```python
from build123d import *

# Parameters (mm, degrees)
F1_DEPTH = 6


with BuildPart() as f1:
    # F0 (on Right) → F1 (new body)
    with BuildSketch(Plane.YZ):
        Polygon((62.5, 142.2184194922), (9.4337919727, 142.2184194922), (9.4337919727, 134.7184194922), (47.5, 134.7184194922), (47.5, 129.8368871212), (62.5, 129.8368871212), align=None)
        Polygon((9.4337919727, 142.2184194922), (-47.5, 142.2184194922), (-47.5, -47.7815805078), (62.5, -47.7815805078), (62.5, 129.8368871212), (47.5, 129.8368871212), (47.5, 114.7184194922), (-32.5, 114.7184194922), (-32.5, 134.7184194922), (9.4337919727, 134.7184194922), align=None)
        Polygon((-22.5, -4.2815805078), (-22.5, -7.7815805078), (-22.5, -11.2815805078), (-32.5, -11.2815805078), (-32.5, -4.2815805078), align=None, mode=Mode.SUBTRACT)
        Polygon((12.5, -4.2815805078), (12.5, -7.7815805078), (12.5, -11.2815805078), (2.5, -11.2815805078), (2.5, -7.7815805078), (2.5, -4.2815805078), align=None, mode=Mode.SUBTRACT)
        Polygon((37.5, -7.7815805078), (37.5, -4.2815805078), (47.5, -4.2815805078), (47.5, -11.2815805078), (37.5, -11.2815805078), align=None, mode=Mode.SUBTRACT)
        Polygon((-22.5, 55.7184194922), (-22.5, 52.2184194922), (-22.5, 48.7184194922), (-32.5, 48.7184194922), (-32.5, 55.7184194922), align=None, mode=Mode.SUBTRACT)
        Polygon((-22.5, 101.2184194922), (-22.5, 97.7184194922), (-32.5, 97.7184194922), (-32.5, 104.7184194922), (-22.5, 104.7184194922), align=None, mode=Mode.SUBTRACT)
        Polygon((12.5, 55.7184194922), (12.5, 52.2184194922), (12.5, 48.7184194922), (2.5, 48.7184194922), (2.5, 52.2184194922), (2.5, 55.7184194922), align=None, mode=Mode.SUBTRACT)
        Polygon((37.5, 52.2184194922), (37.5, 55.7184194922), (47.5, 55.7184194922), (47.5, 48.7184194922), (37.5, 48.7184194922), align=None, mode=Mode.SUBTRACT)
        Polygon((2.5, 97.7184194922), (2.5, 101.2184194922), (2.5, 104.7184194922), (12.5, 104.7184194922), (12.5, 101.2184194922), (12.5, 97.7184194922), align=None, mode=Mode.SUBTRACT)
        Polygon((37.5, 97.7184194922), (37.5, 101.2184194922), (37.5, 104.7184194922), (47.5, 104.7184194922), (47.5, 97.7184194922), align=None, mode=Mode.SUBTRACT)
    extrude(amount=F1_DEPTH)


solid = f1.part
```
For this review, take the finished solid that the model builds, in its own axes (mm). A direction names the side the tool comes from. Round coordinates to 2 decimals unless told otherwise and drop trailing zeros. Loops run counter-clockwise (first coordinate to the right, second up) from the corner with the lowest first, then second, coordinate; pieces in that order, holes last.
(1) We need section A-A (z = 52.5). Give the boundary of the cut face in (x, y).
Returned:
outline: (0, -47.5) - (6, -47.5) - (6, -32.5) - (0, -32.5) - close; (0, -22.5) - (6, -22.5) - (6, 2.5) - (0, 2.5) - close; (0, 12.5) - (6, 12.5) - (6, 37.5) - (0, 37.5) - close; (0, 47.5) - (6, 47.5) - (6, 62.5) - (0, 62.5) - close
(2) We need section C-C (x = 3.65). State how many separate pieces and enclosed holes the cut face has, plus the area to 3 significant figures.
Returned:
separate pieces: 1
enclosed holes: 10
area: 18,700 mm2
(3) Mouldability with a two-part tool opening along Z and no side actions: class faces 3 (the flat face through (3, 8, 142.218)), 4 (the flat face through (3, 37.5, -8)), 5 (the flat face through (0, 6.7, 48.5)) as released by +Z, released by -Z, zero draft, split by the parting line, or undercut.
Returned:
face 3: released by +Z
face 4: undercut
face 5: zero draft
(4) We need section B-B (z = 124). Give the boundary of the cut face in (x, y), plus the area to 3 significant figures.
Returned:
outline: (0, -47.5) - (6, -47.5) - (6, -32.5) - (0, -32.5) - close; (0, 47.5) - (6, 47.5) - (6, 62.5) - (0, 62.5) - close
area: 180 mm2
(5) Wall thickness on line 1 along Z through (x, y) = (2.6, 8.5); line 2 along Y through (x, z) = (3.9, 98); line 3 along Z through (x, y) = (1.35, -20): over which ranges is each line inside the solid? List them lowest first.
Returned:
line 1: z = -47.78 to -11.28, -4.28 to 48.72, 55.72 to 97.72, 104.72 to 114.72, 134.72 to 142.22
line 2: y = -47.5 to -32.5, -22.5 to 2.5, 12.5 to 37.5, 47.5 to 62.5
line 3: z = -47.78 to 114.72, 134.72 to 142.22
(6) Tool access review of faces 1 (the flat face through (3, -32.5, 52)), 2 (the flat face through (3, 7, -47.782)): name each direction out of +Z, -Z, +X, -X, +Y, -Y from which nothing blocks a thin tool from reaching the whole face with its end or side.
Returned:
face 1: +X, -X
face 2: -Z, +X, -X, +Y, -Y
